from build123d import *

# Parameters (mm, degrees)
SKETCH1_W                    = 90
SKETCH1_H                    = 90
BASE_FLANGE1_DEPTH           = 2
EDGE_FLANGE1_STRIP_W         = 9.4732
EDGE_FLANGE1_STRIP_H         = 2
EDGE_FLANGE1_STRIP_CUT_DEPTH = 90
EDGE_FLANGE1_DEPTH           = 90
EDGE_FLANGE3_STRIP_W         = 9.4732
EDGE_FLANGE3_STRIP_H         = 2
EDGE_FLANGE3_STRIP_CUT_DEPTH = 90
EDGE_FLANGE3_DEPTH           = 90
EDGE_FLANGE5_STRIP_CUT_DEPTH = 84.5268
EDGE_FLANGE5_DEPTH           = 84.5268
SKETCH25_W                   = 25
SKETCH25_H                   = 24
CUT_EXTRUDE1_DEPTH           = 119.937769086
SKETCH26_R                   = 5
CUT_EXTRUDE2_DEPTH           = 119.937769086


# Sheet-metal steps are written as plain solids
with BuildPart() as part:
    # Sketch1 → Base-Flange1 (new body)
    with BuildSketch(Plane(origin=(0, 0, 0), x_dir=(1, 0, 0), z_dir=(0, 1, 0))):
        with Locations((2.680250784, -1.97492163)):
            Rectangle(SKETCH1_W, SKETCH1_H)
    extrude(amount=-BASE_FLANGE1_DEPTH)

    # Edge-Flange1 strip (across the edge) → Edge-Flange1 strip cut (cut)
    with BuildSketch(Plane(origin=(-42.319749216, -2, 46.97492163), x_dir=(1, 0, 0), z_dir=(0, 0, -1))):
        with Locations((-2, -1)):
            Rectangle(EDGE_FLANGE1_STRIP_W, EDGE_FLANGE1_STRIP_H)
    extrude(amount=EDGE_FLANGE1_STRIP_CUT_DEPTH, mode=Mode.SUBTRACT)

    # Edge-Flange1 section (across the edge) → Edge-Flange1 (add)
    with BuildSketch(Plane(origin=(-42.319749216, -2, 46.97492163), x_dir=(1, 0, 0), z_dir=(0, 0, -1))):
        with BuildLine():
            Line((0, 0.7366), (0, 38))
            Line((0, 38), (2, 38))
            Line((2, 38), (2, 0.7366))
            ThreePointArc((2, 0.7366), (2.215745145, 0.215745145), (2.7366, 0))
            Line((2.7366, 0), (2.7366, -2))
            ThreePointArc((2.7366, -2), (0.801531583, -1.198468417), (0, 0.7366))
        make_face()
    extrude(amount=EDGE_FLANGE1_DEPTH)

    # Edge-Flange3 strip (across the edge) → Edge-Flange3 strip cut (cut)
    with BuildSketch(Plane(origin=(47.680250784, -2, -43.02507837), x_dir=(-1, 0, 0), z_dir=(0, 0, 1))):
        with Locations((-2, -1)):
            Rectangle(EDGE_FLANGE3_STRIP_W, EDGE_FLANGE3_STRIP_H)
    extrude(amount=EDGE_FLANGE3_STRIP_CUT_DEPTH, mode=Mode.SUBTRACT)

    # Edge-Flange3 section (across the edge) → Edge-Flange3 (add)
    with BuildSketch(Plane(origin=(47.680250784, -2, -43.02507837), x_dir=(-1, 0, 0), z_dir=(0, 0, 1))):
        with BuildLine():
            Line((0, 0.7366), (0, 38))
            Line((0, 38), (2, 38))
            Line((2, 38), (2, 0.7366))
            ThreePointArc((2, 0.7366), (2.215745145, 0.215745145), (2.7366, 0))
            Line((2.7366, 0), (2.7366, -2))
            ThreePointArc((2.7366, -2), (0.801531583, -1.198468417), (0, 0.7366))
        make_face()
    extrude(amount=EDGE_FLANGE3_DEPTH)

    # Edge-Flange5 strip (across the edge) → Edge-Flange5 strip cut (cut)
    with BuildSketch(Plane(origin=(-39.583149216, -2, -43.02507837), x_dir=(0, -0.5000000000000041, 0.8660254037844364), z_dir=(1, 0, 0))):
        Polygon((-8.835731855, 2.791911088), (-0.6317, -1.944688912), (0.3683, -0.212638104), (-7.835731855, 4.523961896), align=None)
    extrude(amount=EDGE_FLANGE5_STRIP_CUT_DEPTH, mode=Mode.SUBTRACT)

    # Edge-Flange5 section (across the edge) → Edge-Flange5 (add)
    with BuildSketch(Plane(origin=(-39.583149216, -2, -43.02507837), x_dir=(0, -0.5000000000000041, 0.8660254037844364), z_dir=(1, 0, 0))):
        with BuildLine():
            Line((-2, 0.425276208), (-2, 43.845299462))
            Line((-2, 43.845299462), (0, 43.845299462))
            Line((0, 43.845299462), (0, 0.425276208))
            ThreePointArc((0, 0.425276208), (0.098685688, 0.056976208), (0.3683, -0.212638104))
            Line((0.3683, -0.212638104), (-0.6317, -1.944688912))
            ThreePointArc((-0.6317, -1.944688912), (-1.63336512, -0.943023792), (-2, 0.425276208))
        make_face()
    extrude(amount=EDGE_FLANGE5_DEPTH)

    # Sketch25 → Cut-Extrude1 (cut, through all)
    with BuildSketch(Plane(origin=(47.680250784, 0, 0), x_dir=(0, 0, -1), z_dir=(1, 0, 0))):
        with Locations((-21.47492163, -28)):
            Rectangle(SKETCH25_W, SKETCH25_H)
    extrude(amount=-CUT_EXTRUDE1_DEPTH, mode=Mode.SUBTRACT)

    # Sketch26 → Cut-Extrude2 (cut, through all)
    with BuildSketch(Plane.ZY.offset(42.319749216)):
        with Locations(Location((-28.02507837, -25, 0), (0, 0, 270))):
            Circle(SKETCH26_R)
    extrude(amount=-CUT_EXTRUDE2_DEPTH, mode=Mode.SUBTRACT)


solid = part.part
For this review, take the finished solid that the model builds, in its own axes (mm). A direction names the side the tool comes from. Round coordinates to 2 decimals unless told otherwise and drop trailing zeros. Loops run counter-clockwise (first coordinate to the right, second up) from the corner with the lowest first, then second, coordinate; pieces in that order, holes last. Notation, with made-up numbers: (23.5, -3) - (69.5, -3) arc R17 ccw to (69.5, 24) - close; hole circle Ø7 at (72, 1.25). An arc over 180 degrees is marked (long way). One line per question, with ' | ' between items.
Q1. The part is to be moulded in two halves that separate along X. For faces 4 (the cylindrical face through (-41.497, -0.78, 2.605)), 5 (the cylindrical face through (-41.334, -21.032, -31.068)), 6 (the flat face through (-40.32, -17, 3)), say which applies: released by +X, released by -X, zero draft, split by the parting line, or undercut.
Taken from the geometry:
face 4: released by -X | face 5: zero draft | face 6: undercut
Q2. For pin 1 (10 mm diameter, centred on x = -14.5, y = -22, fed in from +Z); pin 2 (6 mm diameter, centred on x = -27.5, y = -6, fed in from -Z); pin 3 (10 mm diameter, centred on x = -11, z = -16.5, fed in from -Y), all flat-tipped, find the tip position at first contact; note any pin that passes through.
Taken from the geometry:
pin 1: stops at z = -51.69 | pin 2: stops at z = -49.38 | pin 3: stops at y = -2
Q3. Take a section at D-D (y = -25). Give the boundary of the cut face in (x, z).
Taken from the geometry:
outline: (-42.32, -43.03) - (-40.32, -43.03) - (-40.32, -33.03) - (-42.32, -33.03) - close; (-42.32, -23.03) - (-40.32, -23.03) - (-40.32, 8.97) - (-42.32, 8.97) - close; (-42.32, 33.97) - (-40.32, 33.97) - (-40.32, 46.97) - (-42.32, 46.97) - close; (-39.58, -58.61) - (44.94, -58.61) - (44.94, -56.3) - (-39.58, -56.3) - close; (45.68, -43.03) - (47.68, -43.03) - (47.68, -33.03) - (45.68, -33.03) - close; (45.68, -23.03) - (47.68, -23.03) - (47.68, 8.97) - (45.68, 8.97) - close; (45.68, 33.97) - (47.68, 33.97) - (47.68, 46.97) - (45.68, 46.97) - close
Q4. Take a section at B-B (y = -18). Give the boundary of the cut face in (x, z), and give its area (3 significant figures).
Taken from the geometry:
outline: (-42.32, -43.03) - (-40.32, -43.03) - (-40.32, 8.97) - (-42.32, 8.97) - close; (-42.32, 33.97) - (-40.32, 33.97) - (-40.32, 46.97) - (-42.32, 46.97) - close; (-39.58, -54.57) - (44.94, -54.57) - (44.94, -52.26) - (-39.58, -52.26) - close; (45.68, -43.03) - (47.68, -43.03) - (47.68, 8.97) - (45.68, 8.97) - close; (45.68, 33.97) - (47.68, 33.97) - (47.68, 46.97) - (45.68, 46.97) - close | area: 455 mm²
Q5. Take a section at C-C (x = 13.5). Give the boundary of the cut face in (y, z).
Taken from the geometry:
outline: (-39.97, -64.95) - (-38.97, -66.68) - (-1.37, -44.97) arc R2.74 ccw to (0, -42.6) - (0, 46.97) - (-2, 46.97) - (-2, -42.6) arc R0.74 cw to (-2.37, -43.24) - close
Q6. Tool access review of faces 1 (the flat face through (45.68, -17, 1)), 2 (the flat face through (2, -2, 2)), 3 (the flat face through (2.089, -19.907, -55.673)): name each direction out of +Z, -Z, +X, -X, +Y, -Y from which nothing blocks a thin tool from reaching the whole face with its end or side.
Taken from the geometry:
face 1: +Z, -Z, -Y | face 2: +Z, -Y | face 3: -Z, +X, -X, +Y
Q7. For line 1 along Z through (x, y) = (-41, -25); line 2 along X through (y, z) = (-33, -17); line 3 along Y through (x, z) = (-26.5, 28), list the stretches that pass through material, from the lowest coordinate up. Write a range as [from, to].
Taken from the geometry:
line 1: z = [-43.03, -33.03], [-23.03, 8.97], [33.97, 46.97] | line 2: x = [-42.32, -40.32], [45.68, 47.68] | line 3: y = [-2, 0]
Q8. Take a section at A-A (z = 11). Give the boundary of the cut face in (x, y).
Taken from the geometry:
outline: (-42.32, -16) - (-40.32, -16) - (-40.32, -2.74) arc R0.74 cw to (-39.58, -2) - (44.94, -2) arc R0.74 cw to (45.68, -2.74) - (45.68, -16) - (47.68, -16) - (47.68, -2.74) arc R2.74 ccw to (44.94, 0) - (-39.58, 0) arc R2.74 ccw to (-42.32, -2.74) - close
